Can you work these out from the model? Positions are in its coordinate system, mm. A direction names the side the tool comes from. Coordinates: 2 decimals unless noted, no trailing zeros. Loops run counter-clockwise (first coordinate to the right, second up) from the corner with the lowest first, then second, coordinate; pieces in that order, holes last.
```python
from build123d import *

# Parameters (mm, degrees)
ESQUISSE1_W             = 7.8
ESQUISSE1_H             = 10.8
BOSS_EXTRU_1_DEPTH      = 15
ESQUISSE6_R             = 1.05
ENL_V_MAT_EXTRU_2_DEPTH = 21.061904197
ENL_V_MAT_EXTRU_3_DEPTH = 2
ESQUISSE8_R             = 2.5
ENL_V_MAT_EXTRU_4_DEPTH = 11
ESQUISSE9_W             = 7.8
ESQUISSE9_H             = 5
BOSS_EXTRU_2_DEPTH      = 12
ESQUISSE10_W            = 7.8
ESQUISSE10_H            = 5
BOSS_EXTRU_3_DEPTH      = 12
ESQUISSE11_R            = 1.2
ENL_V_MAT_EXTRU_5_DEPTH = 27.089844768
ESQUISSE15_W            = 1
ESQUISSE15_H            = 4.909128789
ENL_V_MAT_EXTRU_6_DEPTH = 29.384502814
ESQUISSE16_R            = 2.5
ENL_V_MAT_EXTRU_7_DEPTH = 2.5
ESQUISSE17_W            = 1
ESQUISSE17_H            = 4.91
ENL_V_MAT_EXTRU_8_DEPTH = 10
CONG_3_R                = 4
CHANFREIN1_SIZE         = 0.5
CHANFREIN2_SIZE         = 0.5
CONG_5_R                = 0.5


with BuildPart() as part:
    # Esquisse1 → Boss.-Extru.1 (new body)
    with BuildSketch(Plane(origin=(0, 0, 0), x_dir=(1, 0, 0), z_dir=(0, 1, 0))):
        with Locations((3.9, 5.4)):
            Rectangle(ESQUISSE1_W, ESQUISSE1_H)
    extrude(amount=BOSS_EXTRU_1_DEPTH)

    # Esquisse6 → Enlèv. mat.-Extru.2 (cut, through all)
    with BuildSketch(Plane.XZ):
        with Locations(Location((3.9, -5.4, 0), (0, 0, 270))):
            Circle(ESQUISSE6_R)
    extrude(amount=-ENL_V_MAT_EXTRU_2_DEPTH, mode=Mode.SUBTRACT)

    # Esquisse7 → Enlèv. mat.-Extru.3 (cut)
    with BuildSketch(Plane.XZ):
        Polygon((3.9, -7.68), (5.874537921, -6.54), (5.874537921, -4.26), (3.9, -3.12), (1.925462079, -4.26), (1.925462079, -6.54), align=None)
    extrude(amount=-ENL_V_MAT_EXTRU_3_DEPTH, mode=Mode.SUBTRACT)

    # Esquisse8 → Enlèv. mat.-Extru.4 (cut)
    with BuildSketch(Plane(origin=(0, 15, 0), x_dir=(1, 0, 0), z_dir=(0, 1, 0))):
        with Locations(Location((3.9, 5.4, 0), (0, 0, 270))):
            Circle(ESQUISSE8_R)
    extrude(amount=-ENL_V_MAT_EXTRU_4_DEPTH, mode=Mode.SUBTRACT)

    # Esquisse9 → Boss.-Extru.2 (add)
    with BuildSketch(Plane(origin=(0, 0, -10.8), x_dir=(-1, 0, 0), z_dir=(0, 0, -1))):
        with Locations((-3.9, 12.5)):
            Rectangle(ESQUISSE9_W, ESQUISSE9_H)
    extrude(amount=BOSS_EXTRU_2_DEPTH)

    # Esquisse10 → Boss.-Extru.3 (add)
    with BuildSketch(Plane.XY):
        with Locations((3.9, 12.5)):
            Rectangle(ESQUISSE10_W, ESQUISSE10_H)
    extrude(amount=BOSS_EXTRU_3_DEPTH)

    # Esquisse11 → Enlèv. mat.-Extru.5 (cut, through all)
    with BuildSketch(Plane.XZ.offset(-10)):
        with Locations(Location((3.9, -16.8, 0), (0, 0, 270))):
            Circle(ESQUISSE11_R)
        with Locations(Location((3.9, 6, 0), (0, 0, 270))):
            Circle(ESQUISSE11_R)
    extrude(amount=-ENL_V_MAT_EXTRU_5_DEPTH, mode=Mode.SUBTRACT)

    # Esquisse15 → Enlèv. mat.-Extru.6 (cut, through all)
    with BuildSketch(Plane(origin=(0, 15, 0), x_dir=(1, 0, 0), z_dir=(0, 1, 0))):
        with Locations((3.9, -9.545435605)):
            Rectangle(ESQUISSE15_W, ESQUISSE15_H)
    extrude(amount=-ENL_V_MAT_EXTRU_6_DEPTH, mode=Mode.SUBTRACT)

    # Esquisse16 → Enlèv. mat.-Extru.7 (cut)
    with BuildSketch(Plane(origin=(0, 15, 0), x_dir=(1, 0, 0), z_dir=(0, 1, 0))):
        with Locations(Location((3.9, 16.8, 0), (0, 0, 270))):
            Circle(ESQUISSE16_R)
        with Locations((3.9, -6)):
            Circle(ESQUISSE16_R)
    extrude(amount=-ENL_V_MAT_EXTRU_7_DEPTH, mode=Mode.SUBTRACT)

    # Esquisse17 → Enlèv. mat.-Extru.8 (cut)
    with BuildSketch(Plane(origin=(0, 15, 0), x_dir=(1, 0, 0), z_dir=(0, 1, 0))):
        with Locations((3.9, 20.345)):
            Rectangle(ESQUISSE17_W, ESQUISSE17_H)
    extrude(amount=-ENL_V_MAT_EXTRU_8_DEPTH, mode=Mode.SUBTRACT)

    # Congé3
    # the kernel refuses this fillet: 4 mm, written as the material it takes off along each edge
    with BuildSketch(Plane(origin=(7.8, 24.886859967, 12), x_dir=(-1, 0, 0), z_dir=(0, -1, 0)), Plane(origin=(7.8, 0.113140033, -22.8), x_dir=(-1, 0, 0), z_dir=(0, 1, 0))) as cong_3_piece_1:
        with BuildLine():
            CenterArc((4, 3.954743987), CONG_3_R, 180, 81.373073441)
            Line((0, 3.954743987), (-0.08, 3.954743987))
            Line((-0.08, 3.954743987), (-0.08, 0))
            Line((-0.08, 0), (0, -0.08))
            ThreePointArc((0, -0.08), (1.7, -0.08), (3.388, -0.07909488))
            Line((3.388, -0.07909488), (3.4, 0))
        make_face()
    extrude(amount=24.773719933, mode=Mode.SUBTRACT)
    with BuildSketch(Plane(origin=(0, 0.113140033, 12), x_dir=(0, 0, -1), z_dir=(0, 1, 0)), Plane(origin=(0, 24.886859967, -22.8), x_dir=(0, 0, 1), z_dir=(0, -1, 0))) as cong_3_piece_2:
        with BuildLine():
            CenterArc((3.954743987, -4), CONG_3_R, 90, 81.373073441)
            Line((0, -3.4), (-0.07909488, -3.388))
            ThreePointArc((-0.07909488, -3.388), (-0.08, -1.7), (-0.08, 0))
            Line((-0.08, 0), (0, 0.08))
            Line((0, 0.08), (3.954743987, 0.08))
            Line((3.954743987, 0.08), (3.954743987, 0))
        make_face()
    extrude(amount=24.773719933, mode=Mode.SUBTRACT)

    # Chanfrein1
    chanfrein1_edges = [part.edges().sort_by_distance(p)[0] for p in [
        (3.9, 0, -10.8),
        (7.8, 0, -5.4),
        (3.9, 0, 0),
        (0, 0, -5.4),
    ]]
    chamfer(chanfrein1_edges, length=CHANFREIN1_SIZE)

    # Chanfrein2
    chanfrein2_edges = [part.edges().sort_by_distance(p)[0] for p in [
        (0, 5.25, -10.8),
        (7.8, 5.25, -10.8),
        (7.8, 5.25, 0),
        (0, 5.25, 0),
    ]]
    chamfer(chanfrein2_edges, length=CHANFREIN2_SIZE)

    # Congé5
    cong_5_edges = [part.edges().sort_by_distance(p)[0] for p in [
        (0, 15, -5.4),
        (7.8, 15, -5.4),
        (0.966849822, 15, -21.452936975),
        (0.966849822, 15, 10.652936975),
        (6.833150178, 15, -21.452936975),
        (6.833150178, 15, 10.652936975),
    ]]
    fillet(cong_5_edges, radius=CONG_5_R)


solid = part.part
```
(1) If we mould it in two halves opening along X, with no side actions, what happens to faces 6 (the cylindrical face through (0.94, 12.22, 10.62)), 7 (the flat face through (3, 2, -6.4)), 8 (the flat face through (4.87, 0.99, -7.12)), 9 (the flat face through (4, 10, 4))? For each: released by +X, released by -X, zero draft, split by the parting line, or undercut.
Check values:
face 6: released by -X
face 7: undercut
face 8: undercut
face 9: zero draft
(2) If I drill on probe 1 along X at (y, z) = (13, -16.8); probe 2 along X at (y, z) = (2.85, -5.4); probe 3 along Z at (x, y) = (1.75, 12.25), over which ranges is the centre line in solid material (lowest first)?
Check values:
probe 1: x = 0 to 1.4, 6.4 to 7.8
probe 2: x = 0 to 2.85, 4.95 to 7.8
probe 3: z = -22.15 to -6.68, -4.12 to 11.35
(3) Which directions (+Z, -Z, +X, -X, +Y, -Y) give clear straight access to the entire face, cutting with the end or side of a thin tool? Please do faces 1 (the flat face through (3.4, 13, 10)), 2 (the flat face through (2.93, 0.99, -3.68)), 3 (the flat face through (4.4, 13, -21)), 4 (the cylindrical face through (3.8, 13.8, -14.3)), 5 (the flat face through (4, 5, 0)).
Check values:
face 1: +Z, +Y, -Y
face 2: -Y
face 3: -Z, +Y, -Y
face 4: +Y
face 5: +Z, +X, -X, -Y
(4) I'm going to push flat-ended pins straight in: pin 1 (1 mm diameter, centred on x = 3, z = -15, fed in from -Y); pin 2 (4 mm diameter, centred on y = 13, z = -21.5, fed in from -X); pin 3 (4 mm diameter, centred on x = 6, y = 3.5, fed in from -Z); pin 4 (1.7 mm diameter, centred on x = 3.9, z = -5.4, fed in from +Y). Where does each tip first touch, or does it pass through?
Check values:
pin 1: stops at y = 10
pin 2: stops at x = 0.05
pin 3: stops at z = -10.8
pin 4: passes through
(5) I want a section at D-D on y = 11.75. Write out the boundary of the cut face in (x, z).
Check values:
outline: (0, -18.85) arc R4 ccw to (3.4, -22.8) - (3.4, -17.89) arc R1.2 cw (long way) to (4.4, -17.89) - (4.4, -22.8) arc R4 ccw to (7.8, -18.85) - (7.8, 8.05) arc R4 ccw to (4.4, 12) - (4.4, 7.09) arc R1.2 cw (long way) to (3.4, 7.09) - (3.4, 12) arc R4 ccw to (0, 8.05) - close; hole circle Ø5 at (3.9, -5.4)
(6) I want a section at A-A on z = 6. Write out the boundary of the cut face in (x, y).
Check values:
outline: (0, 10) - (2.7, 10) - (2.7, 12.5) - (1.4, 12.5) - (1.4, 15) - (0.5, 15) arc R0.5 ccw to (0, 14.5) - close; (5.1, 10) - (7.8, 10) - (7.8, 14.5) arc R0.5 ccw to (7.3, 15) - (6.4, 15) - (6.4, 12.5) - (5.1, 12.5) - close
(7) I want a section at B-B on y = 4.5. Write out the boundary of the cut face in (x, z), then the cut area to 3 significant figures.
Check values:
outline: (0, -10.3) - (0.5, -10.8) - (7.3, -10.8) - (7.8, -10.3) - (7.8, -0.5) - (7.3, 0) - (0.5, 0) - (0, -0.5) - close; hole circle Ø5 at (3.9, -5.4)
area: 64.1 mm2
(8) I want a section at C-C on z = -5.4. Write out the boundary of the cut face in (x, y).
Check values:
outline: (0, 0.5) - (0.5, 0) - (1.93, 0) - (1.93, 2) - (2.85, 2) - (2.85, 4) - (1.4, 4) - (1.4, 15) - (0.5, 15) arc R0.5 ccw to (0, 14.5) - close; (4.95, 2) - (5.87, 2) - (5.87, 0) - (7.3, 0) - (7.8, 0.5) - (7.8, 14.5) arc R0.5 ccw to (7.3, 15) - (6.4, 15) - (6.4, 4) - (4.95, 4) - close
